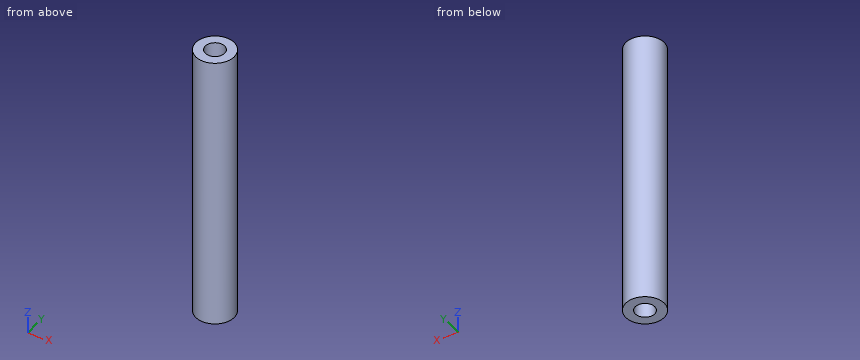
Autodesk Inventor part; units mm, degrees
ref_plane "YZ Plane" through (0, 0, 0) normal (1, 0, 0) x (0, 1, 0)
ref_plane "XZ Plane" through (0, 0, 0) normal (0, 1, 0) x (-1, 0, 0)
ref_plane "XY Plane" through (0, 0, 0) normal (0, 0, 1) x (1, 0, 0)
sketch "Sketch1" plane through (0, 0, 0) normal (0, 0, 1) x (1, 0, 0)
  circle A0 centre (-19.5853, 0.9985) radius 3.1623
  dimension "d0" = 6.3246
extrude "Extrusion1" add sketch "Sketch1" against normal blind 45.8724
sketch "Sketch2" plane through (-19.5853, 0.9985, 0) normal (0, 0, 1) x (1, 0, 0)
  circle A0 centre (0, 0) radius 3.1623
  circle A1 centre (0, 0) radius 1.6002
  dimension "d3" = 3.2004
extrude "Extrusion2" cut sketch "Sketch2" against normal blind 6.35 contours A1
sketch "Sketch3" plane through (-19.5853, 0.9985, -45.8724) normal (0, 0, -1) x (-1, 0, 0)
  circle A0 centre (0, 0) radius 3.1623
  circle A1 centre (0, 0) radius 1.6002
  dimension "d6" = 3.2004
extrude "Extrusion3" cut sketch "Sketch3" against normal blind 6.35 contours A1
properties part number "Roller Axle V4 1764" material "Steel, High Strength Low Alloy"
Read the model definition and answer for the solid it produces. Units are mm, in the model's axes. Coordinates: 2 decimals unless noted, no trailing zeros. Write each loop counter-clockwise with the first axis right and the second up, starting at its lowest first coordinate (ties: lowest second). Pieces come first, ordered by that corner, then holes. Notation, with made-up numbers: (-7, 37.25) - (40, 37.25) arc R30 cw to (40, 76.25) - close; hole circle Ø1 at (24, -17.75). An arc over 180 degrees is marked (long way). Answer as a JSON object with one key per item and string values. Group by question number.
1. A cutting plane is placed at C-C (z = -38). Determine the outline of the cut face in (x, y).
2. Each of these flat-tipped pins is pushed along its axis until it touches: P1, Ø1.6, axis at x = -19.5, y = 0.5, coming from the +Z side; P2, Ø1, axis at x = -20.5, y = 1.5, coming from the -Z side. Where does it stop, or does it pass through?
3. Consider L1, parallel to X at y = 1, z = -43.5; L2, parallel to Z at x = -20.5, y = 1.5; L3, parallel to X at y = 0.75, z = -13. Determine where each line is inside the solid, lowest interval first. Write a range as [from, to].
4. A cutting plane is placed at B-B (y = 0.25). Determine the outline of the cut face in (x, z).
5. A cutting plane is placed at D-D (x = -17.5). Determine the outline of the cut face in (y, z).
6. A cutting plane is placed at A-A (x = -20.5). Determine the outline of the cut face in (y, z), plus the area to 3 significant figures.
Worked out:
{
 "1": {"outline": "circle Ø6.32 at (-19.59, 1)"},
 "2": {"P1": "stops at z = -6.35", "P2": "stops at z = -39.52"},
 "3": {"L1": "x = [-22.75, -21.19], [-17.99, -16.42]", "L2": "z = [-39.52, -6.35]", "L3": "x = [-22.74, -16.43]"},
 "4": {"outline": "(-22.66, -45.87) - (-21, -45.87) - (-21, -39.52) - (-18.17, -39.52) - (-18.17, -45.87) - (-16.51, -45.87) - (-16.51, 0) - (-18.17, 0) - (-18.17, -6.35) - (-21, -6.35) - (-21, 0) - (-22.66, 0) - close"},
 "5": {"outline": "(-1.38, -45.87) - (3.38, -45.87) - (3.38, 0) - (-1.38, 0) - close"},
 "6": {"outline": "(-2.03, -45.87) - (-0.31, -45.87) - (-0.31, -39.52) - (2.31, -39.52) - (2.31, -45.87) - (4.03, -45.87) - (4.03, 0) - (2.31, 0) - (2.31, -6.35) - (-0.31, -6.35) - (-0.31, 0) - (-2.03, 0) - close", "area": "244 mm²"}
}
